Can you work these out from the model? Positions are in its coordinate system, mm. Face numbers are marked on the shaded views. A direction names the side the tool comes from. Round coordinates to 2 decimals unless told otherwise and drop trailing zeros. Order: outer loops, then holes, each group sorted by start corner. A loop starts at its lowest first (then second) coordinate and runs counter-clockwise, first axis right, second up. Notation, with made-up numbers: M 87.25,71 L 143.25,71 A23 ccw 143.25,97 Z; hole C 34,-35.75 d11. An arc over 180 degrees is marked long. Answer as CSV lines item,"result". Start each with the question number.
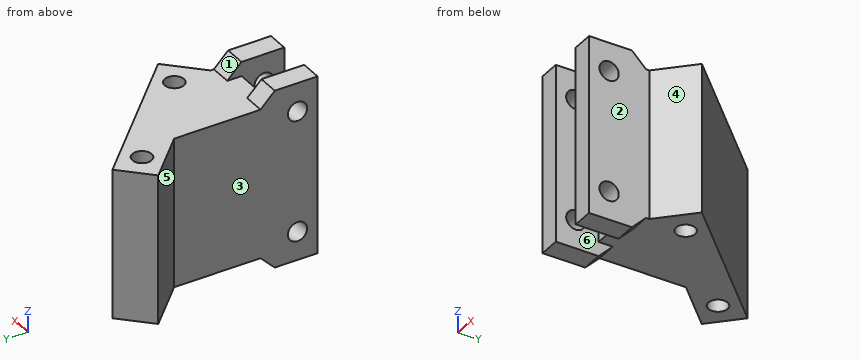
Autodesk Inventor part; units mm, degrees
ref_plane "YZ Plane" through (0, 0, 0) normal (1, 0, 0) x (0, 1, 0)
ref_plane "XZ Plane" through (0, 0, 0) normal (0, 1, 0) x (-1, 0, 0)
ref_plane "XY Plane" through (0, 0, 0) normal (0, 0, 1) x (1, 0, 0)
sketch "Sketch1" plane through (0, 0, 0) normal (0, 0, 1) x (1, 0, 0)
  line L0 (13.7683, -3.4584) -> (10.7683, -3.4584)
  line L1 (13.7683, -3.4584) -> (13.7683, 2.5416)
  circle A0 centre (9.3262, 22.064) radius 1.35
  circle A1 centre (21.3453, 10.0416) radius 1.35
  line L2 (10.7683, -3.4584) -> (13.7683, -3.4584)
  line L3 (9.4532, 26.0885) -> (40.2875, 26.0885) construction
  line L4 (13.7683, 2.5416) -> (18.2683, 2.5416)
  line L5 (10.7683, 16.6612) -> (10.7683, -3.4584)
  line L6 (26.507, 8.8387) -> (-1.0663, 36.4198)
  arc A2 (26.507, 8.8387) -> (30.7497, 8.8382) centre (28.6286, 10.9598) ccw
  line L7 (28.2745, 6.3636) -> (30.7497, 8.8382)
  line L8 (28.2745, 6.3636) -> (20.4257, 7.0011)
  line L9 (20.4257, 7.0011) -> (-6.8649, 34.2993)
  line L10 (-6.8649, 34.2993) -> (-7.5002, 42.1482)
  line L11 (-7.5002, 42.1482) -> (10.4629, 60.1062)
  line L12 (10.4629, 60.1062) -> (18.3117, 59.4687)
  line L13 (18.3117, 59.4687) -> (45.6022, 32.1706)
  line L14 (45.6022, 32.1706) -> (46.2375, 24.3216)
  line L15 (43.7623, 21.8471) -> (46.2375, 24.3216)
  arc A3 (43.7623, 21.8471) -> (43.7628, 26.0897) centre (41.6412, 23.9687) ccw
  line L16 (16.1895, 53.6708) -> (43.7628, 26.0897)
  arc A4 (16.1895, 53.6708) -> (11.9469, 53.6714) centre (14.0679, 51.5497) ccw
  line L17 (-1.0657, 40.6624) -> (11.9469, 53.6714)
  arc A5 (-1.0657, 40.6624) -> (-1.0663, 36.4198) centre (1.0553, 38.5408) ccw
  line L18 (26.507, 8.8387) -> (-1.0663, 36.4198)
  circle A6 centre (18.5232, 55.2968) radius 1.35
  circle A7 centre (-2.693, 34.0865) radius 1.35
  circle A8 centre (9.4722, 55.1566) radius 1.35
  circle A9 centre (30.5424, 43.2743) radius 1.35
  circle A10 centre (42.5615, 31.2518) radius 1.35
  circle A11 centre (-2.5503, 43.1375) radius 1.35
  circle A12 centre (9.3262, 22.064) radius 1.35
  circle A13 centre (21.3453, 10.0416) radius 1.35
  line L19 (4.8715, 22.5596) -> (8.8318, 26.5189)
  line L20 (8.8318, 26.5189) -> (25.8, 9.546)
  line L21 (4.8715, 22.5596) -> (10.7683, 16.6612)
  line L22 (18.2683, -2.9731) -> (18.2683, 2.1519)
  line L23 (18.2683, 2.5416) -> (18.2683, -3.4584)
  line L24 (18.2683, -3.4584) -> (21.2683, -3.4584)
  line L25 (21.2683, -3.4584) -> (21.2683, 5.0155)
  line L26 (25.8, 9.546) -> (21.2683, 5.0155)
  point P0 (0, 0)
  dimension "d9" = 2.7
  dimension "d10" = 2.7
  dimension "d12" = 3
  dimension "d28" = 6
  dimension "d35" = 3.5
  dimension "d36" = 24
  dimension "d38" = 3
  dimension "d63" = 4.5
extrude "Extrusion1" add sketch "Sketch1" along normal blind 25 contours L0 L5 L9 L8 L26 L25 L24 L23 L22 L4 L1 | L9 L19 L6 L26 L8
sketch "Sketch3" plane through (10.7683, -3.4584, 0) normal (-1, 0, 0) x (0, 0, 1)
  circle A0 centre (2, 2.8104) radius 1.35
  circle A1 centre (19, 2.8104) radius 1.35
  line L0 (25, 0) -> (25, 20.1196)
  line L1 (0, 20.1196) -> (0, 0)
  circle A2 centre (4, 2.8104) radius 1.35
  circle A3 centre (21, 2.8104) radius 1.35
  dimension "d48" = 2.7
  dimension "d49" = 2.7
  dimension "d50" = 4
  dimension "d51" = 4
extrude "Extrusion3" cut sketch "Sketch3" against normal through all contours A0 A2 | A0 A2 | A1 A3 | A1 A3 picked at (3.1032, 2.701) picked at (4.6704, 2.7032) picked at (20.1032, 2.9198) picked at (21.6704, 2.9176)
sketch "Sketch5" plane through (10.7683, -3.4584, 0) normal (-1, 0, 0) x (0, 0, 1)
  line L0 (0, 0) -> (25, 0)
  line L1 (0, 0) -> (0, 8.4739)
  line L2 (0, 6) -> (2, 6)
  line L3 (2, 6) -> (2, 32)
  line L4 (2, 32) -> (0, 32)
  line L5 (0, 32) -> (0, 6)
  line L6 (25, 8.4739) -> (25, 0)
  line L7 (25, 6) -> (23, 6)
  line L8 (23, 6) -> (23, 32)
  line L9 (23, 32) -> (25, 32)
  line L10 (25, 32) -> (25, 6)
  point P0 (0, 3.4584)
  dimension "d52" = 2
  dimension "d53" = 26
  dimension "d54" = 6
  dimension "d55" = 2
  dimension "d56" = 26
  dimension "d57" = 6
extrude "Extrusion4" cut sketch "Sketch5" along normal through all both and the other way through all
chamfer "Chamfer1" distance 2 angle 45 4 edges at (12.2683, 2.5416, 23) (19.7683, 2.5416, 23) (19.7683, 2.5416, 2) (12.2683, 2.5416, 2)
properties part number "Knee - Back" material "Aluminum-6061"
(1) I want a section at C-C on z = 4. Write out the boundary of the cut face in (x, y), and give its area (3 significant figures).
(2) If I drill on line 1 along X through (y, z) = (-1.75, 5); line 2 along X through (y, z) = (13, 8.25); line 3 along X through (y, z) = (4.25, 4), over which ranges is the centre line in solid material (lowest first)?
(3) I want a section at D-D on z = 14.75. Write out the boundary of the cut face in (x, y), and give its area (3 significant figures).
(4) I'm going to push flat-ended pins straight in: P1, Ø9, axis at y = 1.5, z = 8, coming from the -X side; P2, Ø6, axis at x = 7.5, z = 7, coming from the -Y side; P3, Ø10.5, axis at x = 19, y = 17, coming from the +Z side; P4, Ø1.6, axis at y = -0.648, z = 4, coming from the -X side. Where does each tip first touch, or does it pass through?
(5) I want a section at B-B on x = 9.5. Write out the boundary of the cut face in (y, z), and give its area (3 significant figures).
(6) For the marked faces 1, 2 and 3, which set-ups out of +Z, -Z, +X, -X, +Y, -Y let a thin tool reach every point of the face, with its end or its side?
(7) I want a section at A-A on y = 21.25. Write out the boundary of the cut face in (x, z), and give its area (3 significant figures).
(8) If we mould it in two halves opening along X, with no side actions, what happens to the marked faces 4, 5 and 6? For each: +X half, -X half, draft (parallel to the pull), parting line (faces both ways), or undercut.
From the geometry:
1,outline,"M 4.87,22.56 L 10.77,16.66 L 10.77,0.7 L 13.77,0.7 L 13.77,2.54 L 18.27,2.54 L 18.27,0.7 L 21.27,0.7 L 21.27,5.02 L 25.8,9.55 L 8.83,26.52 Z; M 10.77,-3.46 L 13.77,-3.46 L 13.77,-2 L 10.77,-2 Z; M 18.27,-3.46 L 21.27,-3.46 L 21.27,-2 L 18.27,-2 Z; hole C 9.33,22.06 d2.7; hole C 21.35,10.04 d2.7"
1,area,"236 mm²"
2,line 1,"10.77 to 13.77, 18.27 to 21.27"
2,line 2,"10.77 to 22.35"
2,line 3,"10.77 to 21.27"
3,outline,"M 4.87,22.56 L 10.77,16.66 L 10.77,-3.46 L 13.77,-3.46 L 13.77,2.54 L 18.27,2.54 L 18.27,-3.46 L 21.27,-3.46 L 21.27,5.02 L 25.8,9.55 L 8.83,26.52 Z; hole C 9.33,22.06 d2.7; hole C 21.35,10.04 d2.7"
3,area,"252 mm²"
4,P1,"x = 10.77"
4,P2,"y = 16.93"
4,P3,"z = 23"
4,P4,"through"
5,outline,"M 17.93,2 L 20.73,2 L 20.73,23 L 17.93,23 Z; M 23.4,2 L 25.85,2 L 25.85,23 L 23.4,23 Z"
5,area,"110 mm²"
6,face 1,"+Z, +X, -X, +Y"
6,face 2,"+Z, -Z, +X, -Y"
6,face 3,"+Z, -Z, -X, -Y"
7,outline,"M 6.18,2 L 8.25,2 L 8.25,23 L 6.18,23 Z; M 10.4,2 L 14.1,2 L 14.1,23 L 10.4,23 Z"
7,area,"121 mm²"
8,face 4,"+X half"
8,face 5,"-X half"
8,face 6,"undercut"
